Autodesk Fusion 360 part; units mm, degrees
sketch "Sketch1" plane through (0, 0, 0) normal (0, 0, 1) x (1, 0, 0)
sketch "Sketch2" plane through (0, 0, 0) normal (0, 0, 1) x (1, 0, 0)
  circle A0 centre (0, 0) radius 3
  dimension "d1" = 6
sketch "Sketch3" plane through (0, 0, 0) normal (0, 1, 0) x (1, 0, 0)
  line L0 (0, 0) -> (0, 17.5)
  line L1 (-7.5, 25) -> (-42.5, 25)
  line L2 (-50, 17.5) -> (-50, 0)
  arc A0 (0, 17.5) -> (-7.5, 25) centre (-7.5, 17.5) ccw
  arc A1 (-42.5, 25) -> (-50, 17.5) centre (-42.5, 17.5) ccw
  point P0 (0, 25)
  point P1 (-50, 25)
  dimension "d2" = 25
  dimension "d4" = 7.5
  dimension "d5" = 7.5
sweep "Sweep1" add profiles "Sketch2" path "Sketch3" along L0 A0 L1 A1 L2 section 1
sketch "Sketch4" plane through (0, 0, 0) normal (0, 0, 1) x (1, 0, 0)
  circle A0 centre (0, 0) radius 1
  dimension "d12" = 2
extrude "Extrude1" cut sketch "Sketch4" against normal blind 15
sketch "Sketch5" plane through (0, 0, 0) normal (0, 0, 1) x (-1, 0, 0)
  circle A0 centre (50, 0) radius 3
  circle A1 centre (50, 0) radius 1
  dimension "d15" = 2
extrude "Extrude2" cut sketch "Sketch5" against normal blind 15 contours A1
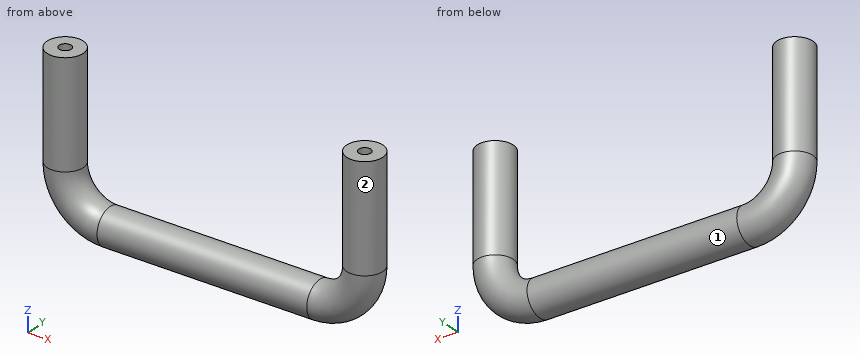
Input: part model. Units: mm. Frame: model coordinates. Face numbers are marked on the shaded views. A direction names the side the tool comes from. Give positions to 0.01 mm unless a question says otherwise; leave off trailing zeros. Write each loop counter-clockwise with the first axis right and the second up, starting at its lowest first coordinate (ties: lowest second). Pieces come first, ordered by that corner, then holes. Notation, with made-up numbers: (44.5, 63) -> (70.5, 63) arc R6 cw to (70.5, 73) -> close; hole circle Ø1 at (28.5, 29.5). An arc over 180 degrees is marked (long way). Use one line per item in the form item = value. Start each with the question number.
1) Pin query (flat end, axial travel): pin 1 (1.6 mm diameter, centred on x = 0, y = 0, fed in from -Z); pin 2 (1 mm diameter, centred on x = -30, y = 2.5, fed in from -Z); pin 3 (1.6 mm diameter, centred on x = -50, y = 0, fed in from +Z); pin 4 (12 mm diameter, centred on x = -40.5, z = -12, fed in from -Y). Return the tip coordinate at first contact, or that it passes through.
2) Section query B-B on y = 0. Return the cut outline in (x, z).
3) Ray query, probe 1 along Y at (x, z) = (-50, -12); probe 2 along X at (y, z) = (-2.5, -21.75); probe 3 along Z at (x, y) = (-23, 0.25). Return the intervals inside material, ascending. Write a range as from..to.
4) Section query C-C on x = -15. Return the cut outline in (y, z).
5) Set-up query: the marked faces 1 and 2. Return all of +Z, -Z, +X, -X, +Y, -Y with unobstructed straight access to the full face (end or side cutting, diameter ignored); none if empty.
6) Section query A-A on z = -8. Return the cut outline in (x, y), then the cut area to 3 significant figures.
Outcome:
q1.pin_1 = -25.58
q1.pin_2 = -27.24
q1.pin_3 = -15
q1.pin_4 = through
q2.outline = (-53, -17.5) arc R10.5 ccw to (-42.5, -28) -> (-7.5, -28) arc R10.5 ccw to (3, -17.5) -> (3, 0) -> (1, 0) -> (1, -15) -> (-1, -15) -> (-1, 0) -> (-3, 0) -> (-3, -17.5) arc R4.5 cw to (-7.5, -22) -> (-42.5, -22) arc R4.5 cw to (-47, -17.5) -> (-47, 0) -> (-49, 0) -> (-49, -15) -> (-51, -15) -> (-51, 0) -> (-53, 0) -> close
q3.probe_1 = -3..-1, 1..3
q3.probe_2 = -50.61..-46.51, -3.49..0.61
q3.probe_3 = -27.99..-22.01
q4.outline = circle Ø6 at (0, -25)
q5.face_1 = none
q5.face_2 = +Z
q6.outline = circle Ø6 at (-50, 0); circle Ø6 at (0, 0); hole circle Ø2 at (-50, 0); hole circle Ø2 at (0, 0)
q6.area = 50.3 mm^2
